Could you check a few things on this model? Use its own coordinates, in mm. A direction names the side the tool comes from. Round coordinates to 2 decimals unless told otherwise and drop trailing zeros. Loops run counter-clockwise (first coordinate to the right, second up) from the corner with the lowest first, then second, coordinate; pieces in that order, holes last. Notation, with made-up numbers: M 8,50.25 L 18,50.25 A8 cw 18,65.25 Z; hole C 67.25,51.5 d2. An arc over 180 degrees is marked long. Answer in a Markdown table with one row per item.
Autodesk Inventor part; units mm, degrees
ref_plane "YZ Plane" through (0, 0, 0) normal (1, 0, 0) x (0, 1, 0)
ref_plane "XZ Plane" through (0, 0, 0) normal (0, 1, 0) x (-1, 0, 0)
ref_plane "XY Plane" through (0, 0, 0) normal (0, 0, 1) x (1, 0, 0)
sketch "Náčrt1" plane through (0, 0, 0) normal (0, 1, 0) x (-1, 0, 0)
  line L0 (24, -47.25) -> (19.6818, -47.25)
  line L1 (24, -47.25) -> (24, -17.0868)
  line L2 (24, -17.0868) -> (49.75, -17.0868)
  line L3 (49.75, 48.4103) -> (49.75, -17.0868)
  line L4 (49.75, 48.4103) -> (-49.75, 48.4103)
  line L5 (-49.75, 48.4103) -> (-49.75, -17.0868)
  line L6 (-24, -17.0868) -> (-49.75, -17.0868)
  line L7 (-24, -47.25) -> (-24, -17.0868)
  line L8 (-19.6818, -47.25) -> (-24, -47.25)
  arc A0 (-18.3182, -47.25) -> (-19.6818, -47.25) centre (-19, -43.5625) ccw
  line L9 (-12, -47.25) -> (-18.3182, -47.25)
  line L10 (-12, -47.25) -> (-12, -40)
  line L11 (-12, -40) -> (-3.25, -40)
  arc A1 (-3, -40.25) -> (-3.25, -40) centre (-3.25, -40.25) ccw
  line L12 (-3, -40.25) -> (-3, -40.6521)
  arc A2 (-3, -40.6521) -> (-2.6294, -40.8711) centre (-2.75, -40.6521) ccw
  arc A3 (2.0811, -47.25) -> (-2.6294, -40.8711) centre (-0.7, -44.375) ccw
  line L13 (18.3182, -47.25) -> (2.0811, -47.25)
  arc A4 (19.6818, -47.25) -> (18.3182, -47.25) centre (19, -43.5625) ccw
  arc A5 (-30.6049, -8.4571) -> (-29.8978, -8.75) centre (-29.8978, -7.75) ccw
  line L14 (-30.6049, -8.4571) -> (-39.25, 0.188)
  line L15 (-39.25, 2.8608) -> (-39.25, 0.188)
  line L16 (-46.25, 2.8608) -> (-39.25, 2.8608)
  ellipse E0 centre (-46.25, 4.3321) end of major axis (-46.25, 2.8608) minor radius 1 (-47.25, 4.3321) -> (-46.25, 2.8608) ccw
  line L17 (-47.25, 4.3321) -> (-47.25, 36.8221)
  arc A6 (-46.25, 37.8221) -> (-47.25, 36.8221) centre (-46.25, 36.8221) ccw
  line L18 (-46.25, 37.8221) -> (-45.25, 37.8221)
  arc A7 (-45.25, 37.8221) -> (-44.25, 38.8221) centre (-45.25, 38.8221) ccw
  line L19 (-44.25, 41.8041) -> (-44.25, 38.8221)
  arc A8 (-36.75, 41.8041) -> (-44.25, 41.8041) centre (-40.5, 41.8041) ccw
  line L20 (-36.75, 38.8221) -> (-36.75, 41.8041)
  arc A9 (-36.75, 38.8221) -> (-35.75, 37.8221) centre (-35.75, 38.8221) ccw
  line L21 (-35.75, 37.8221) -> (-25.4142, 37.8221)
  arc A10 (-24.7071, 37.5292) -> (-25.4142, 37.8221) centre (-25.4142, 36.8221) ccw
  line L22 (-22.7929, 35.615) -> (-24.7071, 37.5292)
  arc A11 (-22.7929, 35.615) -> (-22.0858, 35.3221) centre (-22.0858, 36.3221) ccw
  line L23 (-22.0858, 35.3221) -> (22.0858, 35.3221)
  arc A12 (22.0858, 35.3221) -> (22.7929, 35.615) centre (22.0858, 36.3221) ccw
  line L24 (22.7929, 35.615) -> (24.7071, 37.5292)
  arc A13 (25.4142, 37.8221) -> (24.7071, 37.5292) centre (25.4142, 36.8221) ccw
  line L25 (35.75, 37.8221) -> (25.4142, 37.8221)
  arc A14 (35.75, 37.8221) -> (36.75, 38.8221) centre (35.75, 38.8221) ccw
  line L26 (36.75, 38.8221) -> (36.75, 41.8041)
  arc A15 (44.25, 41.8041) -> (36.75, 41.8041) centre (40.5, 41.8041) ccw
  line L27 (44.25, 41.8041) -> (44.25, 38.8221)
  arc A16 (44.25, 38.8221) -> (45.25, 37.8221) centre (45.25, 38.8221) ccw
  line L28 (46.25, 37.8221) -> (45.25, 37.8221)
  arc A17 (47.25, 36.8221) -> (46.25, 37.8221) centre (46.25, 36.8221) ccw
  line L29 (47.25, 4.3321) -> (47.25, 36.8221)
  ellipse E1 centre (46.25, 4.3321) end of major axis (46.25, 2.8608) minor radius 1 (46.25, 2.8608) -> (47.25, 4.3321) ccw
  line L30 (46.25, 2.8608) -> (39.25, 2.8608)
  line L31 (39.25, 2.8608) -> (39.25, 0.188)
  line L32 (30.6049, -8.4571) -> (39.25, 0.188)
  arc A18 (29.8978, -8.75) -> (30.6049, -8.4571) centre (29.8978, -7.75) ccw
  line L33 (29.8978, -8.75) -> (-29.8978, -8.75)
  line L34 (-3.45, -32.125) -> (-3.45, -26.625)
  line L35 (-3.45, -26.625) -> (2.05, -26.625)
  line L36 (2.05, -26.625) -> (2.05, -32.125)
  line L37 (2.05, -32.125) -> (-3.45, -32.125)
  line L38 (6.3401, -40.3942) -> (9.6599, -40.3942)
  line L39 (9.6599, -40.3942) -> (11.3198, -43.2692)
  line L40 (11.3198, -43.2692) -> (9.6599, -46.1442)
  line L41 (9.6599, -46.1442) -> (6.3401, -46.1442)
  line L42 (6.3401, -46.1442) -> (4.6802, -43.2692)
  line L43 (4.6802, -43.2692) -> (6.3401, -40.3942)
  circle A19 centre (-19, -22.9375) radius 1.75
  circle A20 centre (-20, 39.763) radius 1.75
  circle A21 centre (20, 39.763) radius 1.75
  circle A22 centre (19, -22.9375) radius 1.75
  circle A23 centre (42.25, -8.75) radius 1.75
  circle A24 centre (-42.25, -8.75) radius 1.75
  line L44 (38.75, 0.3951) -> (38.75, 3.3608)
  line L45 (38.75, 3.3608) -> (46.25, 3.3608)
  line L46 (46.75, 4.3321) -> (46.75, 36.8221)
  arc A25 (46.75, 36.8221) -> (46.25, 37.3221) centre (46.25, 36.8221) ccw
  line L47 (46.25, 37.3221) -> (45.25, 37.3221)
  arc A26 (43.75, 38.8221) -> (45.25, 37.3221) centre (45.25, 38.8221) ccw
  line L48 (43.75, 38.8221) -> (43.75, 41.8041)
  arc A27 (43.75, 41.8041) -> (37.25, 41.8041) centre (40.5, 41.8041) ccw
  line L49 (37.25, 41.8041) -> (37.25, 38.8221)
  arc A28 (35.75, 37.3221) -> (37.25, 38.8221) centre (35.75, 38.8221) ccw
  line L50 (35.75, 37.3221) -> (25.4142, 37.3221)
  arc A29 (25.4142, 37.3221) -> (25.0607, 37.1756) centre (25.4142, 36.8221) ccw
  line L51 (25.0607, 37.1756) -> (23.1464, 35.2614)
  arc A30 (22.0858, 34.8221) -> (23.1464, 35.2614) centre (22.0858, 36.3221) ccw
  line L52 (22.0858, 34.8221) -> (-22.0858, 34.8221)
  arc A31 (-23.1464, 35.2614) -> (-22.0858, 34.8221) centre (-22.0858, 36.3221) ccw
  line L53 (-23.1464, 35.2614) -> (-25.0607, 37.1756)
  arc A32 (-25.0607, 37.1756) -> (-25.4142, 37.3221) centre (-25.4142, 36.8221) ccw
  line L54 (-25.4142, 37.3221) -> (-35.75, 37.3221)
  arc A33 (-37.25, 38.8221) -> (-35.75, 37.3221) centre (-35.75, 38.8221) ccw
  line L55 (-37.25, 38.8221) -> (-37.25, 41.8041)
  arc A34 (-37.25, 41.8041) -> (-43.75, 41.8041) centre (-40.5, 41.8041) ccw
  line L56 (-43.75, 41.8041) -> (-43.75, 38.8221)
  arc A35 (-45.25, 37.3221) -> (-43.75, 38.8221) centre (-45.25, 38.8221) ccw
  line L57 (-45.25, 37.3221) -> (-46.25, 37.3221)
  arc A36 (-46.25, 37.3221) -> (-46.75, 36.8221) centre (-46.25, 36.8221) ccw
  line L58 (-46.75, 36.8221) -> (-46.75, 4.3321)
  line L59 (-46.25, 3.3608) -> (-38.75, 3.3608)
  line L60 (-38.75, 3.3608) -> (-38.75, 0.3951)
  line L61 (-38.75, 0.3951) -> (-30.2513, -8.1036)
  arc A37 (-30.2513, -8.1036) -> (-29.8978, -8.25) centre (-29.8978, -7.75) ccw
  line L62 (-29.8978, -8.25) -> (29.8978, -8.25)
  arc A38 (29.8978, -8.25) -> (30.2513, -8.1036) centre (29.8978, -7.75) ccw
  line L63 (30.2513, -8.1036) -> (38.75, 0.3951)
  line L64 (45.25, 37.3221) -> (35.75, 37.3221)
  line L65 (-35.75, 37.3221) -> (-45.25, 37.3221)
  spline S0 degree 5 poles (46.25, 3.3609) (46.281, 3.3609) (46.3118, 3.3675) (46.3409, 3.3802) (46.4606, 3.4487) (46.5476, 3.5625) (46.6014, 3.6535) (46.6833, 3.8417) (46.7286, 4.0407) (46.7429, 4.1374) (46.75, 4.2348) (46.75, 4.3321) knots 0 0 0 0 0 0 0.13219 0.13219 0.13219 0.585181 0.585181 0.585181 1 1 1 1 1 1
  spline S1 degree 5 poles (-46.75, 4.3321) (-46.75, 4.2348) (-46.7429, 4.1374) (-46.7286, 4.0407) (-46.6833, 3.8417) (-46.6014, 3.6535) (-46.5476, 3.5625) (-46.4606, 3.4487) (-46.3409, 3.3802) (-46.3118, 3.3675) (-46.281, 3.3609) (-46.25, 3.3609) knots 0 0 0 0 0 0 0.414819 0.414819 0.414819 0.86781 0.86781 0.86781 1 1 1 1 1 1
  point P0 (0, 0)
  point P1 (0, 0)
  dimension "d0" = 0.5
extrude "Vysunutí1" add sketch "Náčrt1" along normal blind 0.4 contours L63 A38 L62 A37 L61 L60 L59 S1 L58 A36 L57 L65 L54 A32 L53 A31 L52 A30 L51 A29 L50 L64 L47 A25 L46 S0 L45 L44
properties part number "base_plate_isolation"
1) Which directions (+Z, -Z, +X, -X, +Y, -Y) give clear straight access to the entire face, cutting with the end or side of a thin tool? Please do faces 4 (the face through (1, 0.4, 15)), 5 (the face through (-24.117, 0.197, 36.232)).
Computed:
| item | result |
|---|---|
| face 4 | +Z, -Z, +X, -X, +Y |
| face 5 | +Z, +Y, -Y |
2) I want a section at A-A, the plane x = 41.5. Please give me the cut outline in (y, z), plus the area to 3 significant figures.
Computed:
| item | result |
|---|---|
| outline | M 0,3.36 L 0.4,3.36 L 0.4,37.32 L 0,37.32 Z |
| area | 13.6 mm² |
3) If we mould it in two halves opening along X, with no side actions, what happens to faces 1 (the face through (34.56, 0.197, -3.795)), 2 (the face through (24.09, 0.197, 36.205)), 3 (the face through (-34.441, 0.197, -3.914))? For each: released by +X, released by -X, zero draft, split by the parting line, or undercut.
Computed:
| item | result |
|---|---|
| face 1 | released by +X |
| face 2 | undercut |
| face 3 | released by -X |
4) I need wall thicknesses on line 1 (Z direction, x = -15, y = 0.35); line 2 (Z direction, x = 41, y = 0.15); line 3 (X direction, y = 0.3, z = 35.5). Which ranges of each line are inside material? Lowest first, please.
Computed:
| item | result |
|---|---|
| line 1 | z = -8.25 to 34.82 |
| line 2 | z = 3.36 to 37.32 |
| line 3 | x = -46.75 to -23.39, 23.39 to 46.75 |
5) I want a section at B-B, the plane x = 1. Please give me the cut outline in (y, z), plus the area to 3 significant figures.
Computed:
| item | result |
|---|---|
| outline | M 0,-8.25 L 0.4,-8.25 L 0.4,34.82 L 0,34.82 Z |
| area | 17.2 mm² |
